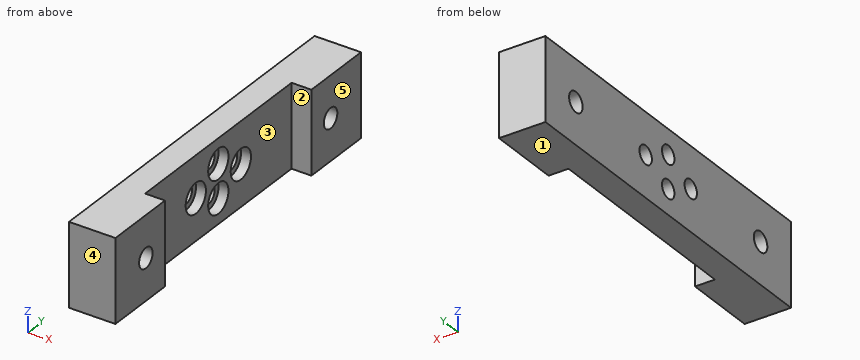
Autodesk Inventor part; units mm, degrees
ref_plane "YZ Plane" through (0, 0, 0) normal (1, 0, 0) x (0, 1, 0)
ref_plane "XZ Plane" through (0, 0, 0) normal (0, 1, 0) x (-1, 0, 0)
ref_plane "XY Plane" through (0, 0, 0) normal (0, 0, 1) x (1, 0, 0)
sketch "Sketch1" plane through (0, 0, 0) normal (0, 1, 0) x (-1, 0, 0)
  line L0 (0, 0) -> (8, 0)
  line L1 (8, 0) -> (8, -25)
  line L2 (8, -25) -> (0, -25)
  line L3 (0, -25) -> (0, 0)
  dimension "d0" = 8
  dimension "d1" = 25
extrude "Extrusion1" add sketch "Sketch1" along normal blind 109
sketch "Sketch2" plane through (0, 0, 0) normal (1, 0, 0) x (0, 0, -1)
  line L0 (0, 109) -> (25, 109)
  line L1 (0, 109) -> (25, 109)
  line L2 (25, 109) -> (25, 87)
  line L3 (25, 87) -> (0, 87)
  line L4 (0, 87) -> (0, 109)
  line L5 (25, 0) -> (25, 109)
  line L6 (25, 0) -> (0, 0)
  line L7 (0, 0) -> (0, 22)
  line L8 (0, 22) -> (25, 22)
  line L9 (25, 22) -> (25, 0)
  dimension "d4" = 25
  dimension "d5" = 22
  dimension "d6" = 25
  dimension "d7" = 22
extrude "Extrusion2" add sketch "Sketch2" along normal blind 6
sketch "Sketch3" plane through (6, 0, 0) normal (1, 0, 0) x (0, 0, -1)
  line L0 (0, 0) -> (25, 0)
  line L1 (0, 0) -> (12.5, 0)
  line L2 (12.5, 0) -> (12.5, 13.5)
  circle A0 centre (12.5, 13.5) radius 3
  circle A1 centre (12.5, 95.5) radius 3
  line L3 (25, 109) -> (0, 109)
  line L4 (0, 109) -> (0, 87)
  dimension "d10" = 13.5
  dimension "d11" = 6
  dimension "d12" = 6
  dimension "d13" = 13.5
  dimension "d14" = 12.5
sketch "Sketch4" plane through (0, 22, -25) normal (1, 0, 0) x (0, 0, -1)
  circle A0 centre (-17.5, 32.5) radius 2.75
  line L0 (-25, -22) -> (0, -22)
  line L1 (-25, 0) -> (-25, 65)
  circle A1 centre (-7.5, 32.5) radius 2.75
  line L2 (0, 0) -> (0, 65)
  circle A2 centre (-12.5, 22.5) radius 2.75
  circle A3 centre (-12.5, 42.5) radius 2.75
  dimension "d15" = 5.5
  dimension "d16" = 54.5
  dimension "d17" = 7.5
  dimension "d18" = 5.5
  dimension "d19" = 7.5
  dimension "d20" = 54.5
  dimension "d21" = 5.5
  dimension "d22" = 5.5
  dimension "d23" = 10
  dimension "d24" = 5
  dimension "d25" = 10
  dimension "d26" = 5
extrude "Extrusion3" cut sketch "Sketch3" against normal up to next
extrude "Extrusion4" cut sketch "Sketch4" against normal up to next
sketch "Sketch5" plane through (0, 22, -25) normal (1, 0, 0) x (0, 0, -1)
  circle A0 centre (-12.5, 42.5) radius 2.75
  circle A1 centre (-12.5, 42.5) radius 4.5
  circle A2 centre (-17.5, 32.5) radius 2.75
  circle A3 centre (-17.5, 32.5) radius 4.5
  circle A4 centre (-7.5, 32.5) radius 2.75
  circle A5 centre (-7.5, 32.5) radius 4.5
  circle A6 centre (-12.5, 22.5) radius 2.75
  circle A7 centre (-12.5, 22.5) radius 4.5
  point P0 (-25, -22)
  dimension "d31" = 9
  dimension "d32" = 9
  dimension "d33" = 9
  dimension "d34" = 9
extrude "Extrusion5" cut sketch "Sketch5" against normal blind 3
properties part number "Back_Bracket" material "ABS Plastic"
Verification items for the finished model (mm, model axes). Face numbers are marked on the shaded views. A direction names the side the tool comes from. Round coordinates to 2 decimals unless told otherwise and drop trailing zeros. Write each loop counter-clockwise with the first axis right and the second up, starting at its lowest first coordinate (ties: lowest second). Pieces come first, ordered by that corner, then holes. Notation, with made-up numbers: (67, 89.5) - (126, 89.5) arc R34 cw to (126, 123.5) - close; hole circle Ø10 at (73.25, -10.5). An arc over 180 degrees is marked (long way). Answer as a JSON object with one key per item and string values. Group by question number.
Q1. Mould release check, pull along Y, two halves, no side actions. Record for the marked faces 3, 4 and 5: released by +Y, released by -Y, zero draft, split by the parting line, or undercut.
Q2. Section check A-A, the plane x = 3.75. Enter the section's corners in (y, z), plus the area to 3 significant figures.
Q3. Section check B-B, the plane y = 44.5. Enter the section's corners in (x, z).
Q4. Thickness scan on line 1 (Y direction, x = -0.5, z = -12.5); line 2 (Y direction, x = -3.5, z = -7.25); line 3 (Z direction, x = 2, y = 11.5). Record the ranges inside material, lowest first.
Q5. Tool access check on the marked faces 1 and 2. Record the directions out of +Z, -Z, +X, -X, +Y, -Y that give a thin tool (end or side, any length) a straight path to the whole face; none if there is none.
Q6. Section check C-C, the plane y = 13.5. Enter the section's corners in (x, z), plus the area to 3 significant figures.
Q7. Go/stop test with flat-tipped pins: pin 1 Ø4 at (x, z) = (-2, -20.5) entering from -Y; pin 2 Ø3 at (y, z) = (43, -7.5) entering from +X; pin 3 Ø4.5 at (y, z) = (66, -14) entering from +X. Record where each tip stops, or that it passes through.
Q8. Section check D-D, the plane y = 79.5. Enter the section's corners in (x, z).
Found:
{
 "1": {"face 3": "undercut", "face 4": "released by -Y", "face 5": "zero draft"},
 "2": {"outline": "(0, -25) - (22, -25) - (22, 0) - (0, 0) - close; (87, -25) - (109, -25) - (109, 0) - (87, 0) - close; hole circle Ø6 at (13.5, -12.5); hole circle Ø6 at (95.5, -12.5)", "area": "1,040 mm^2"},
 "3": {"outline": "(-8, -25) - (0, -25) - (0, -17) - (-3, -17) - (-3, -15.25) - (-8, -15.25) - close; (-8, -9.75) - (-3, -9.75) - (-3, -8) - (0, -8) - (0, 0) - (-8, 0) - close"},
 "4": {"line 1": "y = 0 to 10.5, 16.5 to 40, 49 to 60, 69 to 92.5, 98.5 to 109", "line 2": "y = 0 to 51.76, 57.24 to 109", "line 3": "z = -25 to -14.74, -10.26 to 0"},
 "5": {"face 1": "-Z, +X, -X, +Y, -Y", "face 2": "+Z, -Z, +X"},
 "6": {"outline": "(-8, -25) - (6, -25) - (6, -15.5) - (-8, -15.5) - close; (-8, -9.5) - (6, -9.5) - (6, 0) - (-8, 0) - close", "area": "266 mm^2"},
 "7": {"pin 1": "stops at y = 0", "pin 2": "stops at x = 0", "pin 3": "stops at x = -3"},
 "8": {"outline": "(-8, -25) - (0, -25) - (0, 0) - (-8, 0) - close"}
}
